Source: CAD feature listing. Evaluate the final solid. Frame: model axes, mm. Face numbers are marked on the shaded views. A direction names the side the tool comes from. Round coordinates to 2 decimals unless told otherwise and drop trailing zeros. Write each loop counter-clockwise with the first axis right and the second up, starting at its lowest first coordinate (ties: lowest second). Pieces come first, ordered by that corner, then holes. Notation, with made-up numbers: (11.5, 18) -> (43.5, 18) arc R25 cw to (43.5, 39) -> close; hole circle Ø9 at (67, 47.25). An arc over 180 degrees is marked (long way). Return JSON: item names as keys, results as strings. Group by question number.
from build123d import *

# Parameters (mm, degrees)
BOSS_EXTRUDE1_DEPTH = 8


with BuildPart() as part:
    # Sketch1 → Boss-Extrude1 (new body)
    with BuildSketch(Plane.XY):
        with BuildLine():
            Line((1, 0), (19, 0))
            ThreePointArc((19, 0), (19.707106781, 0.292893219), (20, 1))
            Line((20, 1), (20, 25))
            ThreePointArc((20, 25), (19.707106781, 25.707106781), (19, 26))
            Line((19, 26), (1, 26))
            ThreePointArc((1, 26), (0.292893219, 25.707106781), (0, 25))
            Line((0, 25), (0, 19))
            ThreePointArc((0, 19), (0.292893219, 18.292893219), (1, 18))
            Line((1, 18), (10, 18))
            Line((10, 18), (10, 10))
            Line((10, 10), (1, 10))
            ThreePointArc((1, 10), (0.292893219, 9.707106781), (0, 9))
            Line((0, 9), (0, 1))
            ThreePointArc((0, 1), (0.292893219, 0.292893219), (1, 0))
        make_face()
    extrude(amount=BOSS_EXTRUDE1_DEPTH)


solid = part.part
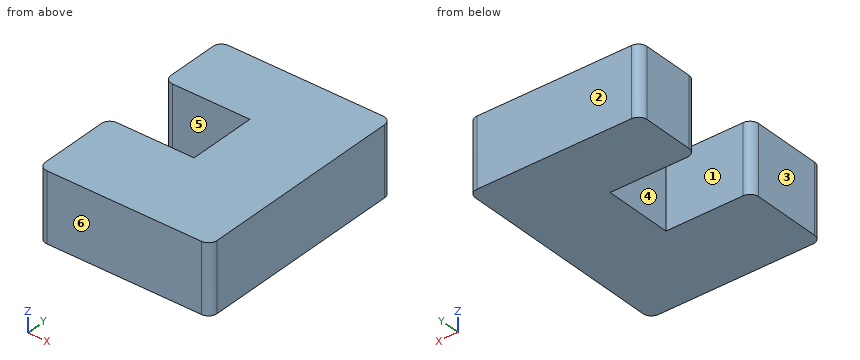
Item 1: Cut plane A-A on x = 9.5. Output: boundary loops of the cut face in (y, z), and give its area (3 significant figures).
Item 2: Cut plane B-B on z = 3.5. Output: boundary loops of the cut face in (x, y), and give its area (3 significant figures).
Item 3: Pull-direction query (Y, two-part tool) for the marked faces 1, 2, 3 and 4; classes: +Y half, -Y half, draft (parallel to the pull), parting line (faces both ways), or undercut.
Item 4: Set-up query: the marked faces 5 and 6. Return all of +Z, -Z, +X, -X, +Y, -Y with unobstructed straight access to the full face (end or side cutting, diameter ignored); none if empty.
Item 5: Material intervals for probe 1 along Y at (x, z) = (1.75, 4); probe 2 along X at (y, z) = (17.25, 5.75); probe 3 along X at (y, z) = (9.5, 3), sorted ascending.
Here are the results:
{
 "1": {"outline": "(0, 0) -> (10, 0) -> (10, 8) -> (0, 8) -> close; (18, 0) -> (26, 0) -> (26, 8) -> (18, 8) -> close", "area": "144 mm^2"},
 "2": {"outline": "(0, 1) arc R1 ccw to (1, 0) -> (19, 0) arc R1 ccw to (20, 1) -> (20, 25) arc R1 ccw to (19, 26) -> (1, 26) arc R1 ccw to (0, 25) -> (0, 19) arc R1 ccw to (1, 18) -> (10, 18) -> (10, 10) -> (1, 10) arc R1 ccw to (0, 9) -> close", "area": "439 mm^2"},
 "3": {"face 1": "undercut", "face 2": "+Y half", "face 3": "draft", "face 4": "undercut"},
 "4": {"face 5": "+Z, -Z, -X", "face 6": "+Z, -Z, +X, -X, -Y"},
 "5": {"probe 1": "y = 0 to 10, 18 to 26", "probe 2": "x = 10 to 20", "probe 3": "x = 0.13 to 20"}
}
